Verification items for the finished model (mm, model axes). A direction names the side the tool comes from. Give positions to 0.01 mm unless a question says otherwise; leave off trailing zeros. Order: outer loops, then holes, each group sorted by start corner. A loop starts at its lowest first (then second) coordinate and runs counter-clockwise, first axis right, second up. Notation, with made-up numbers: (24, 58.5) - (39, 58.5) arc R26 ccw to (39, 73.5) - close; hole circle Ø7 at (57.5, 54). An arc over 180 degrees is marked (long way). Answer as a JSON object with one key per item and string values.
Autodesk Inventor part; units mm, degrees
ref_plane "YZ Plane" through (0, 0, 0) normal (1, 0, 0) x (0, 1, 0)
ref_plane "XZ Plane" through (0, 0, 0) normal (0, 1, 0) x (-1, 0, 0)
ref_plane "XY Plane" through (0, 0, 0) normal (0, 0, 1) x (1, 0, 0)
sketch "Sketch1" plane through (0, 0, 0) normal (0, 1, 0) x (-1, 0, 0)
  line L0 (7.6204, 7.8637) -> (-30.4796, 7.8637)
  line L1 (-30.4796, 7.8637) -> (-30.4796, -49.2863)
  line L2 (-30.4796, -49.2863) -> (-11.4296, -49.2863)
  line L3 (-11.4296, -49.2863) -> (-11.4296, -30.2363)
  line L4 (-11.4296, -30.2363) -> (7.6204, -30.2363)
  line L5 (7.6204, -30.2363) -> (7.6204, 7.8637)
  point P0 (0, 0)
  dimension "d0" = 38.1
  dimension "d1" = 57.15
  dimension "d2" = 19.05
  dimension "d3" = 19.05
  dimension "d4" = 19.05
extrude "Extrusion1" add sketch "Sketch1" along normal blind 19.05
sketch "Sketch2" plane through (0, 19.05, 0) normal (0, 1, 0) x (1, 0, 0)
  line L0 (11.4296, 11.1711) -> (11.4296, -7.8637)
  line L1 (-7.6204, -7.8637) -> (30.4796, -7.8637)
  line L2 (11.4296, 11.1711) -> (30.4796, 11.1711)
  line L3 (30.4796, -7.8637) -> (30.4796, 49.2863)
  line L4 (30.4796, 11.1711) -> (30.4796, -7.8637)
  line L5 (30.4796, -7.8637) -> (11.4296, -7.8637)
  point P0 (0, 0)
extrude "Extrusion2" add sketch "Sketch2" along normal blind 19.05
properties part number "Additive Method(1)"
(1) Section check C-C (x = 6.5). Record the cut outline in (y, z).
Computed values:
{"outline": "(0, -30.24) - (19.05, -30.24) - (19.05, 7.86) - (0, 7.86) - close"}
(2) Section check D-D (z = -35). Record the cut outline in (x, y), then the cut area to 3 significant figures.
Computed values:
{"outline": "(11.43, 0) - (30.48, 0) - (30.48, 19.05) - (11.43, 19.05) - close", "area": "363 mm²"}
(3) Access from +Z, -Z, +X, -X, +Y, -Y to the whole of each face (thin tool, end or side, straight path). Record for faces 1 (the flat face through (21, 28, -11.171)), 2 (the flat face through (21, 9, -49.286)), 3 (the flat face through (2, 9, -30.236)), 4 (the flat face through (11.43, 28, -2)).
Computed values:
{"face 1": "-Z, +X, -X, +Y", "face 2": "-Z, +X, -X, +Y, -Y", "face 3": "-Z, -X, +Y, -Y", "face 4": "+Z, -Z, -X, +Y"}
(4) Gauge pin test, flat ends, axial feed: pin 1 Ø9.5 at (y, z) = (32.5, -2.5) entering from -X; pin 2 Ø5.5 at (x, y) = (18.5, 33) entering from -Z; pin 3 Ø21 at (x, y) = (6, 10) entering from -Z; pin 4 Ø4 at (x, z) = (16.5, -18) entering from +Y. Record the tip position at first contact, or that the pin passes through.
Computed values:
{"pin 1": "stops at x = 11.43", "pin 2": "stops at z = -11.17", "pin 3": "stops at z = -49.29", "pin 4": "stops at y = 19.05"}
(5) Material ranges on line 1 along Y through (x, z) = (19.5, -32); line 2 along Z through (x, y) = (20, 21.5); line 3 along X through (y, z) = (2.5, -34), recorded low to high. Write a range as [from, to].
Computed values:
{"line 1": "y = [0, 19.05]", "line 2": "z = [-11.17, 7.86]", "line 3": "x = [11.43, 30.48]"}
(6) Section check A-A (z = -3). Record the cut outline in (x, y), then the cut area to 3 significant figures.
Computed values:
{"outline": "(-7.62, 0) - (30.48, 0) - (30.48, 38.1) - (11.43, 38.1) - (11.43, 19.05) - (-7.62, 19.05) - close", "area": "1,090 mm²"}
(7) Section check B-B (y = 4.5). Record the cut outline in (x, z).
Computed values:
{"outline": "(-7.62, -30.24) - (11.43, -30.24) - (11.43, -49.29) - (30.48, -49.29) - (30.48, 7.86) - (-7.62, 7.86) - close"}
